from build123d import *

# Parameters (mm, degrees)
F0_R     = 152.6
F0_R_2   = 128.6
F1_DEPTH = 304.8
F3_DEPTH = 25.4
F5_DEPTH = 25.4
F6_R     = 6.35
F7_DEPTH = 382


with BuildPart() as f1:
    # F0 (on Front) → F1 (new body)
    with BuildSketch(Plane.XZ):
        Circle(F0_R)
        Circle(F0_R_2, mode=Mode.SUBTRACT)
    extrude(amount=F1_DEPTH)

    # F2 (on face) → F3 (join)
    with BuildSketch(Plane.XZ.offset(304.8)):
        with BuildLine():
            ThreePointArc((12.7, 127.9713639843), (0, 128.6), (-12.7, 127.9713639843))
            Line((-12.7, 127.9713639843), (-12.7, 12.7))
            Line((-12.7, 12.7), (-12.7, -12.7))
            Line((-12.7, -12.7), (-12.7, -127.9713639843))
            ThreePointArc((-12.7, -127.9713639843), (0, -128.6), (12.7, -127.9713639843))
            Line((12.7, -127.9713639843), (12.7, -12.7))
            Line((12.7, -12.7), (12.7, 12.7))
            Line((12.7, 12.7), (12.7, 127.9713639843))
        make_face()
        with BuildLine():
            Line((-12.7, -12.7), (-12.7, 12.7))
            Line((-12.7, 12.7), (-127.9713639843, 12.7))
            ThreePointArc((-127.9713639843, 12.7), (-128.6, 0), (-127.9713639843, -12.7))
            Line((-127.9713639843, -12.7), (-12.7, -12.7))
        make_face()
        with BuildLine():
            Line((127.9713639843, 12.7), (12.7, 12.7))
            Line((12.7, 12.7), (12.7, -12.7))
            Line((12.7, -12.7), (127.9713639843, -12.7))
            ThreePointArc((127.9713639843, -12.7), (128.6, 0), (127.9713639843, 12.7))
        make_face()
        with BuildLine():
            Line((127.9713639843, 12.7), (12.7, 12.7))
            Line((12.7, 12.7), (12.7, -12.7))
            Line((12.7, -12.7), (127.9713639843, -12.7))
            ThreePointArc((127.9713639843, -12.7), (128.4427448484, -6.3577744384), (128.6, 0))
            ThreePointArc((128.6, 0), (128.4427448484, 6.3577744384), (127.9713639843, 12.7))
        make_face()
    extrude(amount=-F3_DEPTH)

    # F4 (on face) → F5 (join)
    with BuildSketch(Plane(origin=(0, 0, 0), x_dir=(-1, 0, 0), z_dir=(0, 1, 0))):
        with BuildLine():
            Line((-12.7, 127.9713639843), (-12.7, 12.7))
            Line((-12.7, 12.7), (-127.9713639843, 12.7))
            ThreePointArc((-127.9713639843, 12.7), (-128.6, 0), (-127.9713639843, -12.7))
            Line((-127.9713639843, -12.7), (-12.7, -12.7))
            Line((-12.7, -12.7), (-12.7, -127.9713639843))
            ThreePointArc((-12.7, -127.9713639843), (0, -128.6), (12.7, -127.9713639843))
            Line((12.7, -127.9713639843), (12.7, -12.7))
            Line((12.7, -12.7), (127.9713639843, -12.7))
            ThreePointArc((127.9713639843, -12.7), (128.4427448484, -6.3577744384), (128.6, 0))
            ThreePointArc((128.6, 0), (128.4427448484, 6.3577744384), (127.9713639843, 12.7))
            Line((127.9713639843, 12.7), (12.7, 12.7))
            Line((12.7, 12.7), (12.7, 127.9713639843))
            ThreePointArc((12.7, 127.9713639843), (0, 128.6), (-12.7, 127.9713639843))
        make_face()
    extrude(amount=-F5_DEPTH)

    # F6 (on face) → F7 (cut)
    with BuildSketch(Plane(origin=(0, 0, 0), x_dir=(-1, 0, 0), z_dir=(0, 1, 0))):
        Circle(F6_R)
    extrude(amount=-F7_DEPTH, mode=Mode.SUBTRACT)


solid = f1.part
Input: part model. Units: mm. Frame: model coordinates. A direction names the side the tool comes from. Give positions to 0.01 mm unless a question says otherwise; leave off trailing zeros. Order: outer loops, then holes, each group sorted by start corner. A loop starts at its lowest first (then second) coordinate and runs counter-clockwise, first axis right, second up. Notation, with made-up numbers: (-29, -2.5) - (-18, -2.5) arc R24 cw to (-18, 26.5) - close; hole circle Ø7 at (37, 50.25). An arc over 180 degrees is marked (long way). Answer as a JSON object with one key per item and string values. Group by question number.
Q1. Cut plane B-B, the plane z = 0. Output: boundary loops of the cut face in (x, y).
Q2. Line query: probe 1 along Y at (x, z) = (-16.5, 4.5); probe 2 along Z at (x, y) = (0, -139); probe 3 along X at (y, z) = (-288, -116). Output: solid intervals per line, ascending.
Q3. First-contact query: pin 1 Ø3 at (x, y) = (27, -165.5) entering from -Z; pin 2 Ø7.5 at (x, y) = (50.5, -289.5) entering from -Z; pin 3 Ø4 at (y, z) = (-207.5, -15.5) entering from -X. Flat tips, straight axial feed; report the tip coordinate or a pass-through.
Q4. Cut plane D-D, the plane z = 74.5. Output: boundary loops of the cut face in (x, y).
Q5. Cut plane A-A, the plane x = 0. Output: boundary loops of the cut face in (y, z), then the cut area to 3 significant figures.
Q6. Set-up query: faces 1 (the face through (71, -292, 12.7)), 2 (the face through (1, -25.4, 10)). Return all of +Z, -Z, +X, -X, +Y, -Y with unobstructed straight access to the full face (end or side cutting, diameter ignored); none if empty.
Q7. Mould query, pull axis Z, two halves, no side actions, for faces 3 (the face through (-19.87, -150.27, 151.3)), 4 (the face through (12.7, -13, -70)). Classes: pulls with the +Z half, pulls with the -Z half, needs draft (parallel to the pull), parting line crosses it, or undercut.
Q8. Cut plane C-C, the plane x = 69.5. Output: boundary loops of the cut face in (y, z).
Results:
{
 "1": {"outline": "(-152.6, -304.8) - (-6.35, -304.8) - (-6.35, -279.4) - (-128.6, -279.4) - (-128.6, -25.4) - (-6.35, -25.4) - (-6.35, 0) - (-152.6, 0) - close; (6.35, -304.8) - (152.6, -304.8) - (152.6, 0) - (6.35, 0) - (6.35, -25.4) - (128.6, -25.4) - (128.6, -279.4) - (6.35, -279.4) - close"},
 "2": {"probe 1": "-304.8 to -279.4, -25.4 to 0", "probe 2": "-152.6 to -128.6, 128.6 to 152.6", "probe 3": "-99.15 to -55.52, -12.7 to 12.7, 55.52 to 99.15"},
 "3": {"pin 1": "z = -150.45", "pin 2": "z = -145.26", "pin 3": "x = -152"},
 "4": {"outline": "(-133.18, -304.8) - (-104.82, -304.8) - (-104.82, 0) - (-133.18, 0) - close; (-12.7, -304.8) - (12.7, -304.8) - (12.7, -279.4) - (-12.7, -279.4) - close; (-12.7, -25.4) - (12.7, -25.4) - (12.7, 0) - (-12.7, 0) - close; (104.82, -304.8) - (133.18, -304.8) - (133.18, 0) - (104.82, 0) - close"},
 "5": {"outline": "(-304.8, -152.6) - (0, -152.6) - (0, -6.35) - (-25.4, -6.35) - (-25.4, -128.6) - (-279.4, -128.6) - (-279.4, -6.35) - (-304.8, -6.35) - close; (-304.8, 6.35) - (-279.4, 6.35) - (-279.4, 128.6) - (-25.4, 128.6) - (-25.4, 6.35) - (0, 6.35) - (0, 152.6) - (-304.8, 152.6) - close", "area": "27,100 mm^2"},
 "6": {"face 1": "+Y, -Y", "face 2": "none"},
 "7": {"face 3": "parting line crosses it", "face 4": "undercut"},
 "8": {"outline": "(-304.8, -135.85) - (0, -135.85) - (0, -108.2) - (-304.8, -108.2) - close; (-304.8, -12.7) - (-279.4, -12.7) - (-279.4, 12.7) - (-304.8, 12.7) - close; (-304.8, 108.2) - (0, 108.2) - (0, 135.85) - (-304.8, 135.85) - close; (-25.4, -12.7) - (0, -12.7) - (0, 12.7) - (-25.4, 12.7) - close"}
}
